from build123d import *

# Parameters (mm, degrees)
SKETCH1_W                                         = 12.7635
SKETCH1_H                                         = 28.067000578
BOSS_EXTRUDE1_DEPTH                               = 0.762
SKETCH3_W                                         = 12.7635
SKETCH3_H                                         = 28.067000578
BOSS_EXTRUDE2_DEPTH                               = 3.175
CSK_FOR_2_FLAT_HEAD_MACHINE_SCREW_100_D           = 2.7051
CSK_FOR_2_FLAT_HEAD_MACHINE_SCREW_100_DEPTH       = 3.937
CSK_FOR_2_FLAT_HEAD_MACHINE_SCREW_100_CSINK_D     = 4.3688
CSK_FOR_2_FLAT_HEAD_MACHINE_SCREW_100_CSINK_ANGLE = 100
F_16_0_177_DIAMETER_HOLE1_D                       = 4.4958
F_16_0_177_DIAMETER_HOLE1_DEPTH                   = 3.175
CHAMFER1_SIZE                                     = 1.27


with BuildPart() as part:
    # Sketch1 → Boss-Extrude1 (new body)
    with BuildSketch(Plane.XY):
        with Locations((-14.669644351, 41.878697202)):
            Rectangle(SKETCH1_W, SKETCH1_H)
        with BuildLine():
            Line((-9.049894351, 33.115696913), (-9.049894351, 50.641696913))
            ThreePointArc((-9.049894351, 50.641696913), (-9.198684106, 51.000907158), (-9.557894351, 51.149696913))
            Line((-9.557894351, 51.149696913), (-19.781394351, 51.149696913))
            ThreePointArc((-19.781394351, 51.149696913), (-20.140604596, 51.000907158), (-20.289394351, 50.641696913))
            Line((-20.289394351, 50.641696913), (-20.289394351, 33.115696913))
            ThreePointArc((-20.289394351, 33.115696913), (-20.140604596, 32.756486668), (-19.781394351, 32.607696913))
            Line((-19.781394351, 32.607696913), (-9.557894351, 32.607696913))
            ThreePointArc((-9.557894351, 32.607696913), (-9.198684106, 32.756486668), (-9.049894351, 33.115696913))
        make_face(mode=Mode.SUBTRACT)
    extrude(amount=-BOSS_EXTRUDE1_DEPTH)

    # Sketch3 → Boss-Extrude2 (add)
    with BuildSketch(Plane.XY):
        with Locations((-14.669644351, 41.878697202)):
            Rectangle(SKETCH3_W, SKETCH3_H)
    extrude(amount=BOSS_EXTRUDE2_DEPTH)

    # CSK for #2 Flat Head Machine Screw (100)1
    with Locations(Plane(origin=(0, 0, -0.762), x_dir=(-1, 0, 0), z_dir=(0, 0, -1))):
        with Locations((14.669644351, 53.530947491), (14.669644351, 30.226446913)):
            CounterSinkHole(CSK_FOR_2_FLAT_HEAD_MACHINE_SCREW_100_D / 2, CSK_FOR_2_FLAT_HEAD_MACHINE_SCREW_100_CSINK_D / 2, depth=CSK_FOR_2_FLAT_HEAD_MACHINE_SCREW_100_DEPTH, counter_sink_angle=CSK_FOR_2_FLAT_HEAD_MACHINE_SCREW_100_CSINK_ANGLE)

    # #16 (0.177) Diameter Hole1
    with Locations(Plane(origin=(0, 0, 0), x_dir=(-1, 0, 0), z_dir=(0, 0, -1))):
        with Locations((14.479144351, 36.436086129), (14.479144351, 46.940307697)):
            Hole(F_16_0_177_DIAMETER_HOLE1_D / 2, depth=F_16_0_177_DIAMETER_HOLE1_DEPTH)

    # Chamfer1
    chamfer1_edges = [part.edges().sort_by_distance(p)[0] for p in [
        (-8.287894351, 27.845196913, 1.2065),
        (-21.051394351, 27.845196913, 1.2065),
        (-21.051394351, 55.912197491, 1.2065),
        (-8.287894351, 55.912197491, 1.2065),
    ]]
    chamfer(chamfer1_edges, length=CHAMFER1_SIZE)


solid = part.part
Input: part model. Units: mm. Frame: model coordinates. A direction names the side the tool comes from. Give positions to 0.01 mm unless a question says otherwise; leave off trailing zeros. Order: outer loops, then holes, each group sorted by start corner. A loop starts at its lowest first (then second) coordinate and runs counter-clockwise, first axis right, second up. Notation, with made-up numbers: (86, -10.5) -> (131, -10.5) arc R32 ccw to (131, 25.5) -> close; hole circle Ø4 at (-11.5, 15). An arc over 180 degrees is marked (long way). Use one line per item in the form item = value.
1) Reachability of faces 1 (the flat face through (-15, 55.912, 1)), 2 (the flat face through (-15, 42, 0)) from +Z, -Z, +X, -X, +Y, -Y: full face, straight path, thin tool, end or side. Return the list, or none.
Response values:
face_1 = +Z, -Z, +X, -X, +Y
face_2 = -Z
2) Section A-A, the plane y = 38.25. Return loops of the section in (x, z) (3 decimals), and give its area (3 significant figures).
Response values:
outline = (-21.051, -0.762) -> (-20.289, -0.762) -> (-20.289, 0) -> (-15.807, 0) -> (-15.807, 3.175) -> (-21.051, 3.175) -> close; (-13.151, 0) -> (-9.05, 0) -> (-9.05, -0.762) -> (-8.288, -0.762) -> (-8.288, 3.175) -> (-13.151, 3.175) -> close
area = 33.3 mm^2
3) Line query: probe 1 along Y at (x, z) = (-10.5, -0.6); probe 2 along Y at (x, z) = (-15.25, 2.4); probe 3 along Z at (x, y) = (-17.5, 42.5) (3 decimals). Output: solid intervals per line, ascending.
Response values:
probe_1 = 27.85 to 32.61, 51.15 to 55.91
probe_2 = 27.85 to 29, 31.45 to 34.32, 38.55 to 44.83, 49.05 to 52.31, 54.75 to 55.91
probe_3 = 0 to 3.175
4) Section B-B, the plane x = -10.5. Return loops of the section in (y, z) (3 decimals), and give its area (3 significant figures).
Response values:
outline = (27.845, -0.762) -> (32.608, -0.762) -> (32.608, 0) -> (51.15, 0) -> (51.15, -0.762) -> (55.912, -0.762) -> (55.912, 3.175) -> (27.845, 3.175) -> close
area = 96.4 mm^2
5) Section C-C, the plane y = 41.25. Return loops of the section in (x, z) (3 decimals), and give its area (3 significant figures).
Response values:
outline = (-21.051, -0.762) -> (-20.289, -0.762) -> (-20.289, 0) -> (-9.05, 0) -> (-9.05, -0.762) -> (-8.288, -0.762) -> (-8.288, 3.175) -> (-21.051, 3.175) -> close
area = 41.7 mm^2
6) Mould query, pull axis X, two halves, no side actions, for faces 3 (the flat face through (-15, 27.845, 1)), 4 (the cylindrical face through (-14.966, 44.746, 1.61)), 5 (the flat face through (-8.914, 55.268, 1.234)), 6 (the flat face through (-20.408, 55.286, 1.234)). Classes: pulls with the +X half, pulls with the -X half, needs draft (parallel to the pull), parting line crosses it, or undercut.
Response values:
face_3 = needs draft
face_4 = undercut
face_5 = pulls with the +X half
face_6 = pulls with the -X half
7) Section D-D, the plane x = -13.75. Count the separate pieces of the cut face and the enclosed holes in it, and give its area (3 significant figures).
Response values:
separate_pieces = 5
enclosed_holes = 0
area = 52.3 mm^2
8) First-contact query: pin 1 Ø2.5 at (x, y) = (-14.67, 30.23) entering from +Z; pin 2 Ø3 at (x, y) = (-19.5, 45.5) entering from -Z; pin 3 Ø5.5 at (x, y) = (-14.5, 38.5) entering from -Z. Flat tips, straight axial feed; report the tip coordinate or a pass-through.
Response values:
pin_1 = through
pin_2 = -0.76
pin_3 = 0
